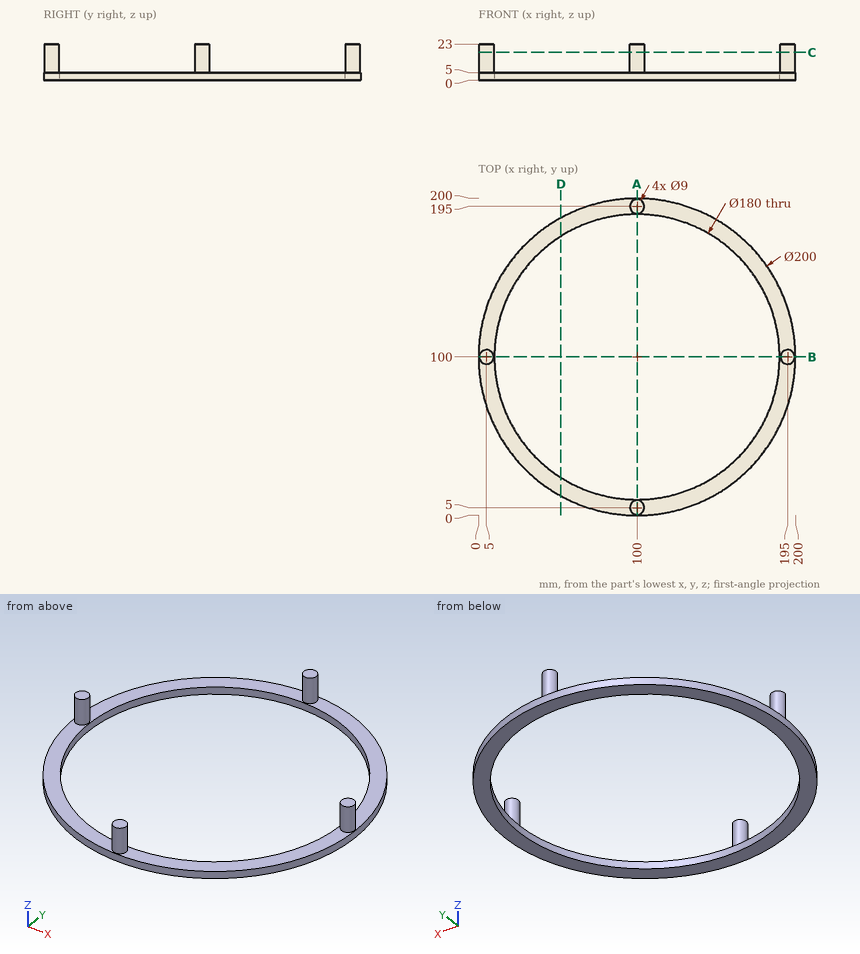
Design review of the part shown in the three views and the two pictorial views. Dimensions are in mm from the part's minimum x, y and z. Round coordinates to 2 decimals unless told otherwise and drop trailing zeros. Loops run counter-clockwise (first coordinate to the right, second up) from the corner with the lowest first, then second, coordinate; pieces in that order, holes last. Notation, with made-up numbers: (41, -38.5) - (45, -38.5) arc R31 cw to (45, -12.5) - close; hole circle Ø6 at (17, 3). An arc over 180 degrees is marked (long way). One line per item, written item: value. Start each with the question number.
Item 1: Take a section at D-D (x = 52). Give the boundary of the cut face in (y, z), plus the area to 3 significant figures.
Item 2: For L1, parallel to Y at x = 100, z = 2.75; L2, parallel to Z at x = 114, y = 192; L3, parallel to Y at x = 58.5, z = 4.75, list the stretches that pass through material, from the lowest coordinate up.
Item 3: Take a section at C-C (z = 17.75). Give the boundary of the cut face in (x, y), plus the area to 3 significant figures.
Item 4: Take a section at A-A (x = 100). Give the boundary of the cut face in (y, z).
Item 5: Clearance check with flat-ended pins moving along their axes: pin 1 Ø3 at (x, z) = (102, 14.5) entering from -Y; pin 2 Ø8 at (x, z) = (48.5, 5) entering from +Y. State where each tip first meets the part, or that it passes through.
Answer below:
1. outline: (12.27, 0) - (23.87, 0) - (23.87, 5) - (12.27, 5) - close; (176.13, 0) - (187.73, 0) - (187.73, 5) - (176.13, 5) - close
1. area: 116 mm2
2. L1: y = 0 to 10, 190 to 200
2. L2: z = 0 to 5
2. L3: y = 9.02 to 20.14, 179.86 to 190.98
3. outline: circle Ø9 at (5, 100); circle Ø9 at (100, 5); circle Ø9 at (100, 195); circle Ø9 at (195, 100)
3. area: 254 mm2
4. outline: (0, 0) - (10, 0) - (10, 5) - (9.5, 5) - (9.5, 23) - (0.5, 23) - (0.5, 5) - (0, 5) - close; (190, 0) - (200, 0) - (200, 5) - (199.5, 5) - (199.5, 23) - (190.5, 23) - (190.5, 5) - (190, 5) - close
5. pin 1: stops at y = 0.53
5. pin 2: stops at y = 188
